Source: CAD feature listing. Evaluate the final solid. Frame: model axes, mm. A direction names the side the tool comes from. Round coordinates to 2 decimals unless told otherwise and drop trailing zeros. Write each loop counter-clockwise with the first axis right and the second up, starting at its lowest first coordinate (ties: lowest second). Pieces come first, ordered by that corner, then holes. Notation, with made-up numbers: (52.5, 62) -> (93.5, 62) arc R30 ccw to (93.5, 95) -> close; hole circle Ø8 at (-7, 11.25). An arc over 180 degrees is marked (long way). Put each result on its own line as item: value.
```python
from build123d import *

# Parameters (mm, degrees)
ESTRUSIONE_ESTRUSIONE1_DEPTH = 5
SCHIZZO2_W                   = 72.109898292
SCHIZZO2_H                   = 42.507089678
ESTRUSIONE_ESTRUSIONE2_DEPTH = 5
SCHIZZO3_W                   = 10.696209694
SCHIZZO3_H                   = 5.348104847
ESTRUSIONE_ESTRUSIONE3_DEPTH = 5
RACCORDO1_R                  = 1.275157777
TAGLIO_ESTRUSIONE1_DEPTH     = 5
SCHIZZO6_W                   = 21.26
SCHIZZO6_H                   = 3
ESTRUSIONE_ESTRUSIONE4_DEPTH = 35
RACCORDO9_DEPTH              = 5
RACCORDO14_R                 = 2
RACCORDO15_R                 = 2


with BuildPart() as part:
    # Schizzo1 → Estrusione-Estrusione1 (new body)
    with BuildSketch(Plane.XY):
        with BuildLine():
            Line((-5.348104847, 0), (-5.348104847, 37.158984831))
            ThreePointArc((-5.348104847, 37.158984831), (0, 42.507089678), (5.348104847, 37.158984831))
            Line((5.348104847, 37.158984831), (5.348104847, 0))
            ThreePointArc((5.348104847, 0), (0, -5.348104847), (-5.348104847, 0))
        make_face()
    extrude(amount=ESTRUSIONE_ESTRUSIONE1_DEPTH)

    # Schizzo2 → Estrusione-Estrusione2 (add)
    with BuildSketch(Plane.XY):
        with Locations((-41.403053993, 21.253544839)):
            Rectangle(SCHIZZO2_W, SCHIZZO2_H)
    extrude(amount=ESTRUSIONE_ESTRUSIONE2_DEPTH)

    # Schizzo3 → Estrusione-Estrusione3 (add)
    with BuildSketch(Plane.XY.offset(5)):
        with Locations((0, 39.833037254)):
            Rectangle(SCHIZZO3_W, SCHIZZO3_H)
    extrude(amount=-ESTRUSIONE_ESTRUSIONE3_DEPTH)

    # Raccordo1
    raccordo1_edges = [part.edges().sort_by_distance(p)[0] for p in [
        (-5.348104847, 0, 2.5),
    ]]
    fillet(raccordo1_edges, radius=RACCORDO1_R)

    # Schizzo5 → Taglio-Estrusione1 (cut)
    with BuildSketch(Plane.XY.offset(5)):
        Polygon((-77.458003139, 21.253544839), (-6.499352309, 0), (-77.458003139, 0), align=None)
    extrude(amount=-TAGLIO_ESTRUSIONE1_DEPTH, mode=Mode.SUBTRACT)

    # Schizzo6 → Estrusione-Estrusione4 (add)
    with BuildSketch(Plane(origin=(0, 0, 0), x_dir=(0, -1, 0), z_dir=(0, 0, -1))):
        with Locations((-31.877089678, 78.958003139)):
            Rectangle(SCHIZZO6_W, SCHIZZO6_H)
    extrude(amount=-ESTRUSIONE_ESTRUSIONE4_DEPTH)

    # Raccordo9: read off the stored shape, not the designer's step
    # Raccordo9 outline → Raccordo9 (add)
    with BuildSketch(Plane.XY):
        with BuildLine():
            ThreePointArc((-78.02262727, 21.247089678), (-77.442645969, 21.204819039), (-76.874922759, 21.078900524))
            Line((-76.874922759, 21.078900524), (-77.458003139, 21.253544839))
            Line((-77.458003139, 21.253544839), (-77.458003139, 21.247089678))
            Line((-77.458003139, 21.247089678), (-78.02262727, 21.247089678))
        make_face()
    extrude(amount=RACCORDO9_DEPTH)

    # Raccordo14
    raccordo14_edges = [part.edges().sort_by_distance(p)[0] for p in [
        (-80.458003139, 31.877089678, 0),
    ]]
    fillet(raccordo14_edges, radius=RACCORDO14_R)

    # Raccordo15
    # the kernel refuses this fillet: 2 mm, written as the material it adds along each edge
    with BuildSketch(Plane(origin=(-77.458003139, 42.507089678, 5), x_dir=(1, 0, 0), z_dir=(0, -1, 0))) as raccordo15_piece_1:
        with BuildLine():
            CenterArc((RACCORDO15_R, RACCORDO15_R), RACCORDO15_R, 180, 90)
            Line((0, RACCORDO15_R), (0, 0))
            Line((0, 0), (RACCORDO15_R, 0))
        make_face()
    extrude(amount=21.253544839)
    with BuildSketch(Plane(origin=(-77.458003139, 21.253544839, 5), x_dir=(1, 0, 0), z_dir=(0, -1, 0))) as raccordo15_piece_2_section:
        with BuildLine():
            CenterArc((RACCORDO15_R, RACCORDO15_R), RACCORDO15_R, 180, 90)
            Line((RACCORDO15_R * 9.50990397541e-11, RACCORDO15_R), (0, 0))
            Line((0, 0), (RACCORDO15_R, 0))
        make_face()
    raccordo15_piece_2 = extrude(amount=5.006455161, mode=Mode.PRIVATE)
    raccordo15_piece_2 = split(raccordo15_piece_2, bisect_by=Plane(origin=(-77.458003139, 21.253544839, 5), z_dir=(0.2869261276439439, 0.957952711398246, 0)), keep=Keep.TOP, mode=Mode.PRIVATE)
    add(raccordo15_piece_2)


solid = part.part
```
Q1. Pin query (flat end, axial travel): pin 1 (3.5 mm diameter, centred on x = -79.5, z = 17, fed in from -Y); pin 2 (14.5 mm diameter, centred on x = -36.5, y = 8, fed in from +Z); pin 3 (2 mm diameter, centred on x = -13.5, y = 27, fed in from -Z); pin 4 (2 mm diameter, centred on y = 26.5, z = 29.5, fed in from +X). Return the tip coordinate at first contact, or that it passes through.
Ans:
pin 1: stops at y = 21.25
pin 2: stops at z = 5
pin 3: stops at z = 0
pin 4: stops at x = -77.46
Q2. Cut plane B-B on z = 8.5. Output: boundary loops of the cut face in (x, y).
Ans:
outline: (-80.46, 21.25) -> (-77.46, 21.25) -> (-77.46, 42.51) -> (-80.46, 42.51) -> close
Q3. Cut plane C-C on x = -48. Output: boundary loops of the cut face in (y, z), and give its area (3 significant figures).
Ans:
outline: (12.43, 0) -> (42.51, 0) -> (42.51, 5) -> (12.43, 5) -> close
area: 150 mm^2
Q4. Material intervals for line 1 (Z direction, x = -30, y = 31.5); line 2 (X direction, y = 22, z = 14.5); line 3 (Y direction, x = -44.5, z = 3), sorted ascending. Write a range as [from, to].
Ans:
line 1: z = [0, 5]
line 2: x = [-80.46, -77.46]
line 3: y = [11.38, 42.51]
Q5. Reachability of faces 1 (the flat face through (-44, 42.507, 3)), 2 (the flat face through (-77.458, 32, 20)) from +Z, -Z, +X, -X, +Y, -Y: full face, straight path, thin tool, end or side. Return the list, or none.
Ans:
face 1: +Z, -Z, +X, -X, +Y
face 2: +Z, +X, +Y, -Y
Q6. Cut plane A-A on y = 36. Output: boundary loops of the cut face in (x, z), and give its area (3 significant figures).
Ans:
outline: (-80.46, 2) arc R2 ccw to (-78.46, 0) -> (5.35, 0) -> (5.35, 5) -> (-75.46, 5) arc R2 cw to (-77.46, 7) -> (-77.46, 35) -> (-80.46, 35) -> close
area: 519 mm^2
